Read the model definition and answer for the solid it produces. Units are mm, in the model's axes. Face numbers are marked on the shaded views. Give positions to 0.01 mm unless a question says otherwise; leave off trailing zeros. Write each loop counter-clockwise with the first axis right and the second up, starting at its lowest first coordinate (ties: lowest second). Pieces come first, ordered by that corner, then holes. Notation, with made-up numbers: (63.25, -10) - (74.25, -10) arc R19 ccw to (74.25, 22) - close; hole circle Ø8 at (-29.5, 6.5). An arc over 180 degrees is marked (long way). Answer as a JSON object with one key per item and string values. Group by question number.
```python
from build123d import *

# Parameters (mm, degrees)
SKETCH2_R          = 1.9812
CUT_EXTRUDE1_DEPTH = 61.53685169
CUT_EXTRUDE2_START = 24.13
SKETCH3_R          = 3.556
CUT_EXTRUDE2_DEPTH = 2.54
CIRPATTERN1_COUNT  = 6


with BuildPart() as part:
    # Sketch1 → Revolve1 (revolve)
    with BuildSketch(Plane(origin=(0, 0, 0), x_dir=(0, 0, -1), z_dir=(1, 0, 0)), mode=Mode.PRIVATE) as revolve1_sk:
        Polygon((0, 23.5077), (27.94, 23.5077), (27.94, 22.225), (46.99, 22.225), (46.99, 23.8125), (28.575, 26.9875), (25.4, 26.9875), (25.4, 25.0952), (0, 25.0952), align=None)
    revolve(revolve1_sk.sketch.rotate(Axis((0, 0, 0), (0, 0, -1)), 90), axis=Axis((0, 0, 0), (0, 0, -1)))

    # Sketch2 → Cut-Extrude1 (cut, through all)
    with BuildSketch(Plane(origin=(0, 0, 0), x_dir=(0, 0, -1), z_dir=(1, 0, 0))):
        with Locations(Location((40.64, 0, 0), (0, 0, 179.999999954))):
            Circle(SKETCH2_R)
    cut_extrude1 = extrude(amount=CUT_EXTRUDE1_DEPTH, mode=Mode.SUBTRACT)

    # Sketch3 → Cut-Extrude2 (cut)
    with BuildSketch(Plane(origin=(0, 0, 0), x_dir=(0, 0, -1), z_dir=(1, 0, 0)).offset(CUT_EXTRUDE2_START)):
        with Locations(Location((40.64, 0, 0), (0, 0, 179.999999954))):
            Circle(SKETCH3_R)
    cut_extrude2 = extrude(amount=CUT_EXTRUDE2_DEPTH, mode=Mode.SUBTRACT)

    # CirPattern1: Cut-Extrude1, Cut-Extrude2 ×6 about axis
    cirpattern1_axis = Axis((0, 0, 0), (0, 0, 1))
    add([cut_extrude1.rotate(cirpattern1_axis, i * 360 / CIRPATTERN1_COUNT) for i in range(1, CIRPATTERN1_COUNT)], mode=Mode.SUBTRACT)
    add([cut_extrude2.rotate(cirpattern1_axis, i * 360 / CIRPATTERN1_COUNT) for i in range(1, CIRPATTERN1_COUNT)], mode=Mode.SUBTRACT)


solid = part.part
```
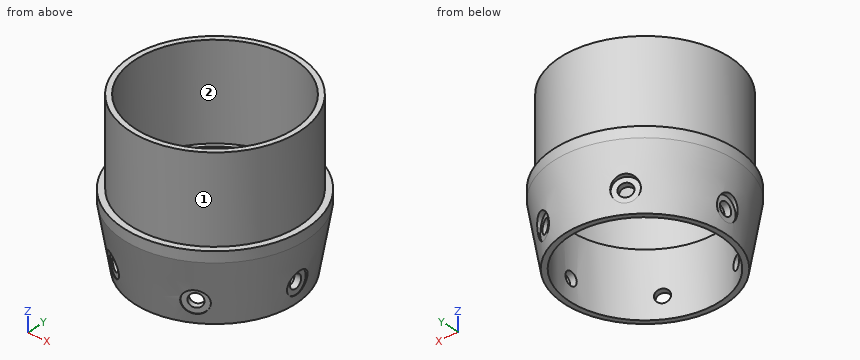
1) Find section A-A, the plane x = 0. Write down the section's boundary in (y, z) (1 decimal).
2) Flat-ended cylindrical pins translate along their axes: pin 1 Ø4.5 at (y, z) = (0, -40.64) entering from -X; pin 2 Ø5 at (x, z) = (12.5, -42) entering from -Y; pin 3 Ø1 at (x, z) = (4.5, -31.5) entering from +Y; pin 4 Ø14 at (x, y) = (11, 10) entering from +Z. Find the tip coordinate at first contact, or state that the pin passes through.
3) For a pull along Y with two mould halves and no side action, classify the marked faces 1 and 2 as released by +Y, released by -Y, zero draft, split by the parting line, or undercut.
4) Find the intervals of material crossed by line 1 (X direction, y = 14.5, z = -22); line 2 (Y direction, x = -9, z = -41.5); line 3 (Y direction, x = -17.5, z = -37.5), in increasing order. Write a range as [from, to].
5) Find section C-C, the plane z = -6.5. Write down the section's boundary in (x, y), and give its area (3 significant figures).
6) Find section B-B, the plane y = 0. Give the number of separate pieces and of enclosed holes in the cut face, and give its area (3 significant figures).
Values follow:
{
 "1": {"outline": "(-27, -28.6) - (-23.8, -47) - (-22.2, -47) - (-22.2, -27.9) - (-23.5, -27.9) - (-23.5, 0) - (-25.1, 0) - (-25.1, -25.4) - (-27, -25.4) - close; (22.2, -47) - (23.8, -47) - (27, -28.6) - (27, -25.4) - (25.1, -25.4) - (25.1, 0) - (23.5, 0) - (23.5, -27.9) - (22.2, -27.9) - close"},
 "2": {"pin 1": "stops at x = -24.13", "pin 2": "stops at y = -22.09", "pin 3": "stops at y = 26.22", "pin 4": "passes through"},
 "3": {"face 1": "split by the parting line", "face 2": "undercut"},
 "4": {"line 1": "x = [-20.48, -18.5], [18.5, 20.48]", "line 2": "y = [-23.07, -20.32], [20.32, 23.07]", "line 3": "y = [-18.48, -13.7], [13.7, 18.48]"},
 "5": {"outline": "circle Ø50.19 at (0, 0); hole circle Ø47.02 at (0, 0)", "area": "242 mm2"},
 "6": {"separate pieces": "4", "enclosed holes": "0", "area": "195 mm2"}
}
